Geometry check sheet. Reference: the model listing, model coordinates, mm. Coordinates: 2 decimals unless noted, no trailing zeros. Loops run counter-clockwise (first coordinate to the right, second up) from the corner with the lowest first, then second, coordinate; pieces in that order, holes last.
from build123d import *

# Parameters (mm, degrees)
SALIENTE_EXTRUIR1_DEPTH = 5
CROQUIS2_W              = 12
CROQUIS2_H              = 150
SALIENTE_EXTRUIR3_DEPTH = 5


with BuildPart() as part:
    # Croquis1 → Saliente-Extruir1 (new body)
    with BuildSketch(Plane(origin=(0, 0, 0), x_dir=(1, 0, 0), z_dir=(0, 1, 0))):
        Polygon((35, 0), (45, 0), (45, 5), (55, 5), (55, 0), (65, 0), (65, 5), (75, 5), (75, 0), (85, 0), (85, 5), (95, 5), (95, 0), (105, 0), (105, 5), (115, 5), (115, 0), (125, 0), (125, 5), (135, 5), (135, 0), (145, 0), (145, 5), (155, 5), (155, 0), (165, 0), (165, 5), (175, 5), (175, 0), (185, 0), (185, 5), (195, 5), (195, 10), (200, 10), (200, 20), (195, 20), (195, 30), (200, 30), (200, 40), (195, 40), (195, 50), (200, 50), (200, 60), (195, 60), (195, 70), (200, 70), (200, 80), (195, 80), (195, 90), (200, 90), (200, 100), (195, 100), (195, 110), (200, 110), (200, 120), (195, 120), (195, 130), (200, 130), (200, 140), (195, 140), (195, 145), (185, 145), (185, 150), (175, 150), (175, 145), (165, 145), (165, 150), (155, 150), (155, 145), (145, 145), (145, 150), (135, 150), (135, 145), (125, 145), (125, 150), (115, 150), (115, 145), (105, 145), (105, 150), (95, 150), (95, 145), (85, 145), (85, 150), (75, 150), (75, 145), (65, 145), (65, 150), (55, 150), (55, 145), (45, 145), (45, 150), (35, 150), (35, 145), (25, 145), (25, 150), (15, 150), (15, 145), (5, 145), (5, 140), (0, 140), (0, 130), (5, 130), (5, 120), (0, 120), (0, 30), (5, 30), (5, 20), (0, 20), (0, 10), (5, 10), (5, 5), (15, 5), (15, 0), (25, 0), (25, 5), (35, 5), align=None)
    extrude(amount=SALIENTE_EXTRUIR1_DEPTH)

    # Croquis2 → Saliente-Extruir3 (add)
    with BuildSketch(Plane(origin=(0, 5, 0), x_dir=(1, 0, 0), z_dir=(0, 1, 0))):
        with Locations((-6, 75)):
            Rectangle(CROQUIS2_W, CROQUIS2_H)
    extrude(amount=-SALIENTE_EXTRUIR3_DEPTH)


solid = part.part
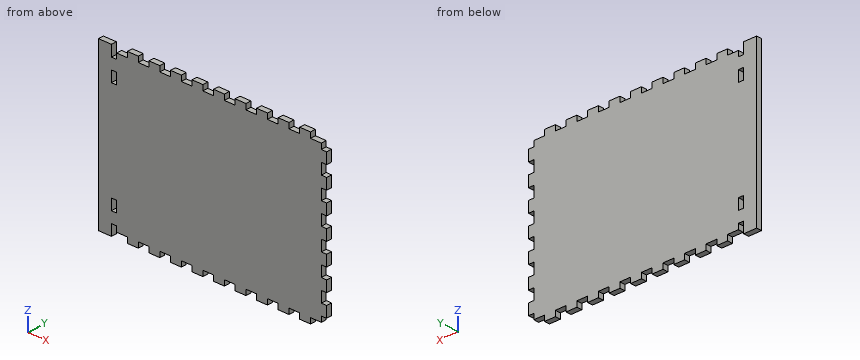
1) Section check B-B on y = 2.9. Count the separate pieces of the cut face and the enclosed holes in it, and give its area (3 significant figures).
Data:
separate pieces: 1
enclosed holes: 2
area: 30,200 mm2
2) Depth check by flat-ended pin: pin 1 (2.5 mm diameter, centred on x = 198.5, y = 1.5, fed in from +Z); pin 2 (2.5 mm diameter, centred on x = 69.5, y = 2.5, fed in from +Z); pin 3 (6 mm diameter, centred on x = 168, z = -120, fed in from -Y); pin 4 (1.5 mm diameter, centred on y = 3.5, z = -127, fed in from +X). Enter the tip coordinate at first touch or a pass-through.
Data:
pin 1: stops at z = -10
pin 2: stops at z = -5
pin 3: stops at y = 0
pin 4: stops at x = 195
3) Section check C-C on x = 92. Record the cut outline in (y, z).
Data:
outline: (0, -145) - (5, -145) - (5, -5) - (0, -5) - close
4) Section check A-A on z = -127. Record the cut outline in (x, y), and give its area (3 significant figures).
Data:
outline: (-12, 0) - (0, 0) - (0, 5) - (-12, 5) - close; (5, 0) - (195, 0) - (195, 5) - (5, 5) - close
area: 1,010 mm2
5) Material ranges on probe 1 along X at (y, z) = (3.7, -125); probe 2 along Z at (x, y) = (131, 1.3); probe 3 along X at (y, z) = (2.05, -83), recorded low to high.
Data:
probe 1: x = -12 to 0, 5 to 195
probe 2: z = -145 to -5
probe 3: x = -12 to 195
6) Section check D-D on z = -67.5. Record the cut outline in (x, y), and give its area (4 significant figures).
Data:
outline: (-12, 0) - (195, 0) - (195, 5) - (-12, 5) - close
area: 1,035 mm2
